Can you work these out from the drawing? Everything is in mm from the part's minimum corner. A direction names the side the tool comes from. Round coordinates to 2 decimals unless told otherwise and drop trailing zeros. Loops run counter-clockwise (first coordinate to the right, second up) from the corner with the lowest first, then second, coordinate; pieces in that order, holes last. Notation, with made-up numbers: (39, 63) -> (58, 63) arc R20 ccw to (58, 88) -> close; hole circle Ø9 at (-0.75, 24.25). An arc over 180 degrees is marked (long way). One line per item, written item: value.
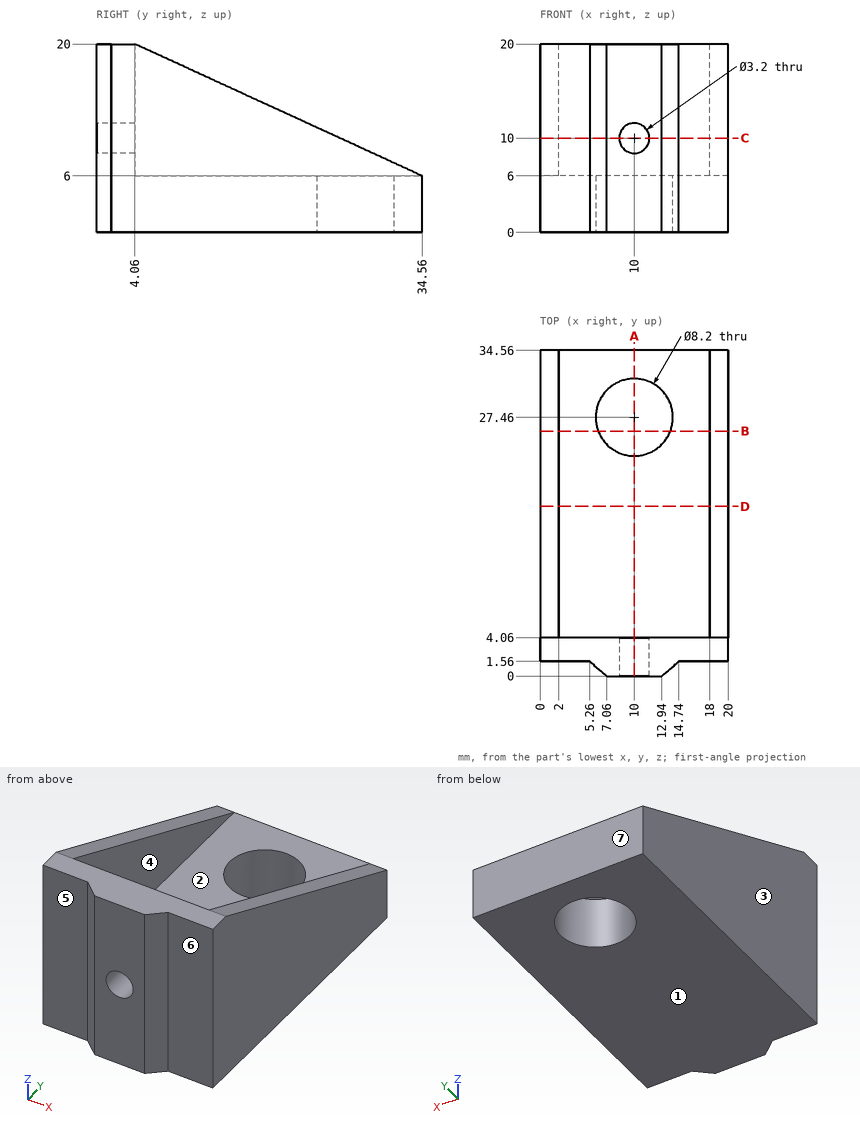
(1) Imagine slicing it at B-B on y = 26. Write out the boundary of the cut face in (x, z), then the cut area to 3 significant figures.
Results below:
outline: (0, 0) -> (6.17, 0) -> (6.17, 6) -> (2, 6) -> (2, 9.93) -> (0, 9.93) -> close; (13.83, 0) -> (20, 0) -> (20, 9.93) -> (18, 9.93) -> (18, 6) -> (13.83, 6) -> close
area: 89.7 mm²
(2) Imagine slicing it at A-A on x = 10. Write out the boundary of the cut face in (y, z), then the cut area to 3 significant figures.
Results below:
outline: (0, 0) -> (23.36, 0) -> (23.36, 6) -> (4.06, 6) -> (4.06, 8.4) -> (0, 8.4) -> close; (0, 11.6) -> (4.06, 11.6) -> (4.06, 20) -> (0, 20) -> close; (31.56, 0) -> (34.56, 0) -> (34.56, 6) -> (31.56, 6) -> close
area: 202 mm²
(3) For pin 1 Ø2.5 at (x, z) = (18, 12) entering from -Y; pin 2 Ø1 at (x, z) = (13.5, 14.5) entering from -Y; pin 3 Ø6 at (x, z) = (3.5, 12) entering from -Y, each with a flat end and sliding along its axis, tell me the tip position at first contact or that it passes through.
Results below:
pin 1: stops at y = 1.56
pin 2: stops at y = 0.05
pin 3: stops at y = 0.49
(4) Imagine slicing it at D-D on y = 18. Write out the boundary of the cut face in (x, z), then the cut area to 3 significant figures.
Results below:
outline: (0, 0) -> (20, 0) -> (20, 13.6) -> (18, 13.6) -> (18, 6) -> (2, 6) -> (2, 13.6) -> (0, 13.6) -> close
area: 150 mm²
(5) On a 3-axis mill with a long thin cutter (end or side, diameter ignored), from which of +Z, -Z, +X, -X, +Y, -Y can I reach the whole of each face in a straight line? I mean the marked faces 4, 5, 6 and 7. Say none if no direction works.
Results below:
face 4: +Z, +Y
face 5: +Z, -Z, -X, -Y
face 6: +Z, -Z, +X, -Y
face 7: +Z, -Z, +X, -X, +Y
(6) Imagine slicing it at C-C on z = 10. Write out the boundary of the cut face in (x, y).
Results below:
outline: (0, 1.56) -> (5.26, 1.56) -> (7.06, 0) -> (8.4, 0) -> (8.4, 4.06) -> (2, 4.06) -> (2, 25.85) -> (0, 25.85) -> close; (11.6, 0) -> (12.94, 0) -> (14.74, 1.56) -> (20, 1.56) -> (20, 25.85) -> (18, 25.85) -> (18, 4.06) -> (11.6, 4.06) -> close
(7) Please list where these lines run through material, in increasing order: L1, parallel to Z at x = 10, y = 1.2; L2, parallel to X at y = 19, z = 7; L3, parallel to Y at x = 10, z = 3.6.
Results below:
L1: z = 0 to 8.4, 11.6 to 20
L2: x = 0 to 2, 18 to 20
L3: y = 0 to 23.36, 31.56 to 34.56
(8) We'd pull the mould along X, two halves only. Please class the marked faces 1, 2 and 3: +X half, -X half, draft (parallel to the pull), parting line (faces both ways), or undercut.
Results below:
face 1: draft
face 2: undercut
face 3: -X half
